Solid Edge part; units mm, degrees
sketch "Sketch1" plane through (0, 0, 0) normal (0, -1, 0) x (1, 0, 0)
  line L0 (-25, -5) -> (25, -5)
  line L1 (25, -5) -> (25, 5)
  line L2 (25, 5) -> (-25, 5)
  line L3 (-25, 5) -> (-25, -5)
  dimension "D1" = 25
extrude "Protrusion1" add sketch "Sketch1" against normal blind 20
sketch "Sketch2" plane through (0, 0, 0) normal (0, -1, 0) x (1, 0, 0)
  circle A0 centre (-20, 0) radius 1.948
  circle A1 centre (20, 0) radius 1.948
extrude "Cutout1" cut sketch "Sketch2" against normal through all
sketch "Sketch3" plane through (0, 0, 0) normal (0, -1, 0) x (1, 0, 0)
  line L0 (-15, 5) -> (15, 5)
  line L1 (15, 5) -> (15, -5)
  line L2 (15, -5) -> (-15, -5)
  line L3 (-15, -5) -> (-15, 5)
extrude "Extrusionsausschnitt_3" cut sketch "Sketch3" against normal blind 15
sketch "Sketch4" plane through (-15, 7.5, 0) normal (1, 0, 0) x (0, 1, 0)
  line L0 (-7.5, 5) -> (-2.5, 5)
  line L1 (-2.5, 5) -> (-2.5, -5)
  line L2 (-2.5, -5) -> (-7.5, -5)
  line L3 (-7.5, -5) -> (-7.5, 5)
  dimension "D1" = 7.5
extrude "Extrusionsausprägung_2" add sketch "Sketch4" along normal blind 30
sketch "Sketch5" plane through (0, 0, 0) normal (0, -1, 0) x (1, 0, 0)
  line L0 (-15, -2.5) -> (-10, -2.5)
  line L1 (-10, -2.5) -> (-10, 2.5)
  line L2 (-10, 2.5) -> (-15, 2.5)
  line L3 (-15, 2.5) -> (-15, -2.5)
  line L4 (15, -2.5) -> (10, -2.5)
  line L5 (10, -2.5) -> (10, 2.5)
  line L6 (10, 2.5) -> (15, 2.5)
  line L7 (15, 2.5) -> (15, -2.5)
  dimension "D1" = 10
extrude "Cutout2" cut sketch "Sketch5" against normal up to next
chamfer "Fase_1" distance 0.5 angle 60 2 edges at (-21.948, 0, 0) (18.052, 0, 0) measured on face at (-16.1667, 0, 3.4333)
properties material "Nylon, allgemein"
Check sheet for the modelled part. Datum: model origin and axes. Units: mm. A direction names the side the tool comes from. Round coordinates to 2 decimals unless told otherwise and drop trailing zeros. Loops run counter-clockwise (first coordinate to the right, second up) from the corner with the lowest first, then second, coordinate; pieces in that order, holes last.
1. Gauge pin test, flat end, axial feed: pin 1 Ø3.5 at (x, z) = (-20, 0) entering from -Y. Record the tip position at first contact, or that the pin passes through.
2. Mould release check, pull along X, two halves, no side actions. Record for faces 5 (the flat face through (25, 10, 0)), 6 (the flat face through (-12, 2, 2.5)), 7 (the flat face through (-10, 2, 0)), 8 (the flat face through (0, 3, -5)): released by +X, released by -X, zero draft, split by the parting line, or undercut.
3. Scan lines: probe 1 along Z at (x, y) = (20, 12.5); probe 2 along Y at (x, z) = (9.5, -1.25); probe 3 along X at (y, z) = (8, -0.75). Record each from-to range of solid material in increasing order.
4. Sectioned sample at C-C on y = 12. Record the boundary of the cut face in (x, z).
5. Sectioned sample at B-B on z = 3.5. Record the boundary of the cut face in (x, y).
6. Sectioned sample at D-D on x = 11.5. Record the boundary of the cut face in (y, z), and give its area (3 significant figures).
7. Set-up check for faces 1 (the flat face through (-15, 9, 0)), 2 (the flat face through (13, 2, -2.5)), 3 (the flat face through (0, 15, 0)), 4 (the flat face through (0, 3, 5)): record each of +Z, -Z, +X, -X, +Y, -Y from which the full face is reachable in a straight line by a thin tool's end or side.
8. Sectioned sample at A-A on x = 1.5. Record the boundary of the cut face in (y, z).
Recorded:
1. pin 1: passes through
2. face 5: released by +X
2. face 6: undercut
2. face 7: undercut
2. face 8: zero draft
3. probe 1: z = -5 to -1.95, 1.95 to 5
3. probe 2: y = 0 to 5, 15 to 20
3. probe 3: x = -25 to -21.8, -18.2 to -15, 15 to 18.2, 21.8 to 25
4. outline: (-25, -5) - (-15, -5) - (-15, 5) - (-25, 5) - close; (15, -5) - (25, -5) - (25, 5) - (15, 5) - close; hole circle Ø3.9 at (-20, 0); hole circle Ø3.9 at (20, 0)
5. outline: (-25, 0) - (25, 0) - (25, 20) - (-25, 20) - close; hole (-15, 5) - (15, 5) - (15, 15) - (-15, 15) - close
6. outline: (0, -5) - (5, -5) - (5, -2.5) - (0, -2.5) - close; (0, 2.5) - (5, 2.5) - (5, 5) - (0, 5) - close; (15, -5) - (20, -5) - (20, 5) - (15, 5) - close
6. area: 75.0 mm2
7. face 1: none
7. face 2: -Y
7. face 3: +Z, -Z
7. face 4: +Z, +X, -X, +Y, -Y
8. outline: (0, -5) - (5, -5) - (5, 5) - (0, 5) - close; (15, -5) - (20, -5) - (20, 5) - (15, 5) - close
